Autodesk Inventor part; units mm, degrees
ref_plane "YZ Plane" through (0, 0, 0) normal (1, 0, 0) x (0, 1, 0)
ref_plane "XZ Plane" through (0, 0, 0) normal (0, 1, 0) x (-1, 0, 0)
ref_plane "XY Plane" through (0, 0, 0) normal (0, 0, 1) x (1, 0, 0)
sketch "Sketch1" plane through (0, 0, 0) normal (1, 0, 0) x (0, 1, 0)
  line L0 (0, 0) -> (661.0386, 0)
  line L1 (661.0386, 0) -> (661.0386, 150)
  line L2 (661.0386, 0) -> (511.0386, 0)
  line L3 (661.0386, 150) -> (586.0386, 150)
  line L4 (586.0386, 150) -> (511.0386, 0)
  point P0 (0, 0)
  dimension "d0" = 150
  dimension "d1" = 150
  dimension "d2" = 75
extrude "Plate1" add sketch "Sketch1" along normal blind 5
sketch "Sketch2" plane through (5, 0, 0) normal (1, 0, 0) x (0, 0, -1)
  line L0 (-150, 661.0386) -> (0, 661.0386)
  line L1 (0, 661.0386) -> (0, 511.0386)
  circle A0 centre (-15, 621.0386) radius 2.5
  line L2 (0, 511.0386) -> (0, 661.0386)
  line L3 (0, 586.0386) -> (-15, 586.0386)
  circle A1 centre (-15, 551.0386) radius 2.5
  point P0 (0, 0)
  dimension "d4" = 40
  dimension "d5" = 15
  dimension "d6" = 5
extrude "Extrusion1" cut sketch "Sketch2" along normal mid plane 10
equation "\"d3\" = Thickness"
equation "\"BendRadius\" = Thickness"
equation "\"BendReliefWidth\" = Thickness"
equation "\"BendReliefDepth\" = 0.5 * Thickness"
equation "\"TransitionRadius\" = BendRadius"
equation "\"JacobiRadiusSize\" = BendRadius"
equation "\"GapSize\" = Thickness"
properties part number "rudder"
Could you check a few things on this model? Use its own coordinates, in mm. Give positions to 0.01 mm unless a question says otherwise; leave off trailing zeros. Write each loop counter-clockwise with the first axis right and the second up, starting at its lowest first coordinate (ties: lowest second). Pieces come first, ordered by that corner, then holes. Notation, with made-up numbers: (-34, 69) -> (22, 69) arc R21 ccw to (22, 95) -> close; hole circle Ø10 at (29, 20). An arc over 180 degrees is marked (long way). Write each question's results on one line, items separated by ' | '. Start each with the question number.
Q1. Suppose I cut it at B-B, the plane x = 1.2. List the corners of the cut face in (y, z) for me.
Q2. Suppose I cut it at D-D, the plane z = 99.5. List the corners of the cut face in (x, y) for me, and give its area (3 significant figures).
Q3. I need wall thicknesses on probe 1 along Y at (x, z) = (3.75, 15); probe 2 along Y at (x, z) = (1, 14.5); probe 3 along Y at (x, z) = (3.95, 114). Which ranges of each line are inside material? Lowest first, please.
Q4. I'm going to push a flat-ended pin straight in: pin 1 Ø12 at (y, z) = (642, 45) entering from -X. Where does the tip first touch, or does it pass through?
Q5. Suppose I cut it at A-A, the plane z = 15. List the corners of the cut face in (x, y) for me.
Q6. Suppose I cut it at C-C, the plane y = 557. List the corners of the cut face in (x, z) for me, and give its area (3 significant figures).
Q7. We'd pull the mould along Y, two halves only. Please class faces 1 (the face through (0, 602, 76)), 2 (the face through (2.54, 623.15, 13.66)), 3 (the face through (2, 661.039, 74)), 4 (the face through (2.465, 549.064, 76.05)): +Y half, -Y half, draft (parallel to the pull), parting line (faces both ways), or undercut.
Outcome:
1) outline: (511.04, 0) -> (661.04, 0) -> (661.04, 150) -> (586.04, 150) -> close; hole circle Ø5 at (551.04, 15); hole circle Ø5 at (621.04, 15)
2) outline: (0, 560.79) -> (5, 560.79) -> (5, 661.04) -> (0, 661.04) -> close | area: 501 mm2
3) probe 1: 518.54 to 548.54, 553.54 to 618.54, 623.54 to 661.04 | probe 2: 518.29 to 548.59, 553.49 to 618.59, 623.49 to 661.04 | probe 3: 568.04 to 661.04
4) pin 1: x = 0
5) outline: (0, 518.54) -> (5, 518.54) -> (5, 548.54) -> (0, 548.54) -> close; (0, 553.54) -> (5, 553.54) -> (5, 618.54) -> (0, 618.54) -> close; (0, 623.54) -> (5, 623.54) -> (5, 661.04) -> (0, 661.04) -> close
6) outline: (0, 0) -> (5, 0) -> (5, 91.92) -> (0, 91.92) -> close | area: 460 mm2
7) face 1: draft | face 2: undercut | face 3: +Y half | face 4: -Y half
